CAD build for the part. Positions are in the model's coordinates, mm. A direction names the side the tool comes from. Round coordinates to 2 decimals unless told otherwise and drop trailing zeros. Loops run counter-clockwise (first coordinate to the right, second up) from the corner with the lowest first, then second, coordinate; pieces in that order, holes last. Notation, with made-up numbers: M 37.25,5 L 91.25,5 A20 ccw 91.25,22 Z; hole C 82.5,66.5 d4. An arc over 180 degrees is marked long. Use one line per item in the form item = value.
from build123d import *

# Parameters (mm, degrees)
SKETCH1_W           = 76
SKETCH1_H           = 35
BOSS_EXTRUDE1_DEPTH = 12
SKETCH4_R           = 3
BOSS_EXTRUDE2_DEPTH = 30
FILLET1_R           = 2


with BuildPart() as part:
    # Sketch1 → Boss-Extrude1 (new body, symmetric)
    with BuildSketch(Plane(origin=(0, 0, 0), x_dir=(1, 0, 0), z_dir=(0, 1, 0))):
        Rectangle(SKETCH1_W, SKETCH1_H)
    extrude(amount=BOSS_EXTRUDE1_DEPTH, both=True)

    # Sketch4 → Boss-Extrude2 (add)
    with BuildSketch(Plane(origin=(-22.75, 0, -22.75), x_dir=(0.707106781, 0, -0.707106781), z_dir=(0.707106781, 0, 0.707106781))):
        with Locations((-9.495689014, 4)):
            Circle(SKETCH4_R)
        with Locations((-9.495689014, -4)):
            Circle(SKETCH4_R)
    extrude(amount=-BOSS_EXTRUDE2_DEPTH)

    # Fillet1
    fillet1_edges = [part.edges().sort_by_distance(p)[0] for p in [
        (-38, 12, 0),
        (0, 12, 17.5),
        (38, 12, 0),
        (0, -12, 17.5),
        (-38, -12, 0),
        (0, -12, -17.5),
        (38, -12, 0),
        (38, 0, 17.5),
        (-38, 0, 17.5),
        (-38, 0, -17.5),
        (38, 0, -17.5),
        (0, 12, -17.5),
    ]]
    fillet(fillet1_edges, radius=FILLET1_R)


solid = part.part
1. Cut at B-B on x = 21.5. Write the cut outline in (y, z).
Completed:
outline = M -12,-15.5 A2 ccw -10,-17.5 L 10,-17.5 A2 ccw 12,-15.5 L 12,15.5 A2 ccw 10,17.5 L -10,17.5 A2 ccw -12,15.5 Z
2. Cut at A-A on z = -7.5. Write the cut outline in (x, y), and give its area (3 significant figures).
Completed:
outline = M -38,-10 A2 ccw -36,-12 L 36,-12 A2 ccw 38,-10 L 38,10 A2 ccw 36,12 L -36,12 A2 ccw -38,10 Z
area = 1,820 mm2
3. Drop flat-ended pins along their axis: P1, Ø4, axis at y = -9.5, z = -1, coming from the -X side; P2, Ø4, axis at y = 5.5, z = -22.5, coming from the +X side. Give the stop position or say it passes through.
Completed:
P1 = -38
P2 = -29.97
4. Probe line 1 along Z through (x, y) = (20.5, 0.5); line 2 along X through (y, z) = (-7.75, 1); line 3 along X through (y, z) = (-3.5, -23.5). List the from-to ranges inside material, lowest first. Write a range as from..to.
Completed:
line_1 = -17.5..17.5
line_2 = -38..38
line_3 = -41.11..-32.75
5. Tool access for faces 4 (the face through (0.5, -11.4, -16.93)), 5 (the face through (-37.4, -0.14, -16.93)): list every direction of +Z, -Z, +X, -X, +Y, -Y with a clear straight run to the whole face (end or side of a thin tool).
Completed:
face_4 = -Z, +X, -X, -Y
face_5 = -X, +Y, -Y
6. Pull direction Y, two halves, no side cores. Call faces 1 (the face through (-38, 0, 0)), 2 (the face through (37.43, 11.4, -0.22)), 3 (the face through (-37.9, -3.1, -28.52)): +Y half, -Y half, draft (parallel to the pull), parting line (faces both ways), or undercut.
Completed:
face_1 = draft
face_2 = +Y half
face_3 = undercut
